```python
from build123d import *

# Parameters (mm, degrees)
F0_R     = 12.7
F0_R_2   = 6.35
F1_DEPTH = 7.62
F0_R_3   = 15.875
F2_DEPTH = 15.24
F3_DEPTH = 27.94
F5_DEPTH = 19.05
F6_DEPTH = 2.54


with BuildPart() as f1:
    # F0 (on Top) → F1 (new body)
    with BuildSketch(Plane.XY):
        Circle(F0_R)
        Circle(F0_R_2, mode=Mode.SUBTRACT)
    extrude(amount=F1_DEPTH)

    # F0 (on Top) → F2 (join)
    with BuildSketch(Plane.XY):
        Circle(F0_R_3)
        Circle(F0_R, mode=Mode.SUBTRACT)
    extrude(amount=F2_DEPTH)

    # F0 (on Top) → F3 (join)
    with BuildSketch(Plane.XY):
        Circle(F0_R_2)
    extrude(amount=F3_DEPTH)

    # F4 (on face) → F5 (join)
    with BuildSketch(Plane.XY.offset(27.94)):
        with BuildLine():
            Line((0, 0), (2.4892, -1.8669))
            ThreePointArc((2.4892, -1.8669), (2.9518280819, -0.983942694), (3.1115, 0))
            ThreePointArc((3.1115, 0), (2.8697186557, 1.2025585587), (2.1819502092, 2.2182257628))
            Line((2.1819502092, 2.2182257628), (0, 0))
        make_face()
        with BuildLine():
            ThreePointArc((2.1819502092, 2.2182257628), (1.6749519392, 2.6222067522), (1.095248, 2.912364))
            Line((1.095248, 2.912364), (0, 0))
            Line((0, 0), (2.1819502092, 2.2182257628))
        make_face()
        with BuildLine():
            ThreePointArc((-2.7755672417, 1.4062925502), (-3.0996598031, -0.2711850936), (-2.4892, -1.8669))
            Line((-2.4892, -1.8669), (0, 0))
            Line((0, 0), (-2.7755672417, 1.4062925502))
        make_face()
        with BuildLine():
            Line((0, 0), (-2.4892, 1.8669))
            ThreePointArc((-2.4892, 1.8669), (-2.6424388986, 1.642847807), (-2.7755672417, 1.4062925502))
            Line((-2.7755672417, 1.4062925502), (0, 0))
        make_face()
        with BuildLine():
            Line((0, 0), (1.095248, 2.912364))
            ThreePointArc((1.095248, 2.912364), (-0.87122, 2.98704), (-2.4892, 1.8669))
            Line((-2.4892, 1.8669), (0, 0))
        make_face()
        with BuildLine():
            ThreePointArc((-2.4892, -1.8669), (0, -3.1115), (2.4892, -1.8669))
            Line((2.4892, -1.8669), (0, 0))
            Line((0, 0), (-2.4892, -1.8669))
        make_face()
    extrude(amount=F5_DEPTH)

    # F4 (on face) → F6 (join)
    with BuildSketch(Plane.XY.offset(27.94)):
        with BuildLine():
            ThreePointArc((-7.2164748284, 3.6563606306), (-8.0591154881, -0.7050812433), (-6.47192, -4.85394))
            Line((-6.47192, -4.85394), (-5.08, -3.81))
            ThreePointArc((-5.08, -3.81), (-6.3258363329, -0.5534389664), (-5.6644229422, 2.8699847964))
            Line((-5.6644229422, 2.8699847964), (-7.2164748284, 3.6563606306))
        make_face()
        with BuildLine():
            Line((-5.08, 3.81), (-6.47192, 4.85394))
            ThreePointArc((-6.47192, 4.85394), (-6.8703411364, 4.2714042983), (-7.2164748284, 3.6563606306))
            Line((-7.2164748284, 3.6563606306), (-5.6644229422, 2.8699847964))
            ThreePointArc((-5.6644229422, 2.8699847964), (-5.3927324462, 3.3527506266), (-5.08, 3.81))
        make_face()
        with BuildLine():
            Line((2.2352, 5.9436), (2.8476448, 7.5721464))
            ThreePointArc((2.8476448, 7.5721464), (-2.265172, 7.766304), (-6.47192, 4.85394))
            Line((-6.47192, 4.85394), (-5.08, 3.81))
            ThreePointArc((-5.08, 3.81), (-1.778, 6.096), (2.2352, 5.9436))
        make_face()
        with BuildLine():
            ThreePointArc((5.6730705438, 5.7673869833), (4.3548750419, 6.8177375558), (2.8476448, 7.5721464))
            Line((2.8476448, 7.5721464), (2.2352, 5.9436))
            ThreePointArc((2.2352, 5.9436), (3.4182692637, 5.3514423515), (4.4529596105, 4.5269913526))
            Line((4.4529596105, 4.5269913526), (5.6730705438, 5.7673869833))
        make_face()
        with BuildLine():
            Line((5.08, -3.81), (6.47192, -4.85394))
            ThreePointArc((6.47192, -4.85394), (7.6747530129, -2.5582510043), (8.0899, 0))
            ThreePointArc((8.0899, 0), (7.4612685048, 3.1266522526), (5.6730705438, 5.7673869833))
            Line((5.6730705438, 5.7673869833), (4.4529596105, 4.5269913526))
            ThreePointArc((4.4529596105, 4.5269913526), (5.8565686851, 2.4542011402), (6.35, 0))
            ThreePointArc((6.35, 0), (6.0241389426, -2.0080463142), (5.08, -3.81))
        make_face()
        with BuildLine():
            ThreePointArc((-6.47192, -4.85394), (0, -8.0899), (6.47192, -4.85394))
            Line((6.47192, -4.85394), (5.08, -3.81))
            ThreePointArc((5.08, -3.81), (0, -6.35), (-5.08, -3.81))
            Line((-5.08, -3.81), (-6.47192, -4.85394))
        make_face()
    extrude(amount=-F6_DEPTH)


solid = f1.part
```
The listing builds one solid part. Answer for the finished solid, in the listing's coordinates (mm). A direction names the side the tool comes from. Round coordinates to 2 decimals unless told otherwise and drop trailing zeros. Loops run counter-clockwise (first coordinate to the right, second up) from the corner with the lowest first, then second, coordinate; pieces in that order, holes last.
Q1. Section C-C, the plane y = 10 is taken. Determine the outline of the cut face in (x, z), then the cut area to 3 significant figures.
Q2. Given pin 1 Ø2 at (x, z) = (6, 10.5) entering from +Y; pin 2 Ø1.5 at (x, z) = (3, 32) entering from -Y; pin 3 Ø4 at (x, y) = (-8.5, -5) entering from -Z; pin 4 Ø1 at (x, y) = (9.5, 7.5) entering from +Z, each flat-ended and moving along its own axis, determine where each tip first touches the part or whether it passes through.
Q3. For a pull along Y with two mould halves and no side action, classify faces 4 (the face through (-3.441, -15.497, 7.513)), 5 (the face through (3, 6, 7.62)), 6 (the face through (0, 0, 46.99)) as released by +Y, released by -Y, zero draft, split by the parting line, or undercut.
Q4. Section A-A, the plane z = 12.5 is taken. Determine the outline of the cut face in (x, y) (3 decimals), then the cut area to 3 significant figures.
Q5. Which of the six approach directions +Z, -Z, +X, -X, +Y, -Y give full straight-line access (tool end or side, diameter ignored) to faces 1 (the face through (0, 0, 0)), 2 (the face through (-2.75, -12.4, 11.38)), 3 (the face through (5.866, -2.432, 16.386))?
Q6. Find the intervals of material crossed by line 1 (Y direction, x = 0, z = 11.5) (3 decimals); line 2 (X direction, y = 4.5, z = 13); line 3 (X direction, y = -5, z = 15), in increasing order.
Q7. Section D-D, the plane z = 37 is taken. Determine the outline of the cut face in (x, y), then the cut area to 3 significant figures.
Completed:
1. outline: (-12.33, 0) - (12.33, 0) - (12.33, 15.24) - (7.83, 15.24) - (7.83, 7.62) - (-7.83, 7.62) - (-7.83, 15.24) - (-12.33, 15.24) - close
1. area: 256 mm2
2. pin 1: stops at y = 15.07
2. pin 2: stops at y = -2.15
2. pin 3: stops at z = 0
2. pin 4: stops at z = 7.62
3. face 4: split by the parting line
3. face 5: undercut
3. face 6: zero draft
4. outline: circle Ø31.75 at (0, 0); circle Ø12.7 at (0, 0); hole circle Ø25.4 at (0, 0)
4. area: 412 mm2
5. face 1: -Z, +X, -X, +Y, -Y
5. face 2: +Z
5. face 3: none
6. line 1: y = -15.875 to -12.7, -6.35 to 6.35, 12.7 to 15.875
6. line 2: x = -15.22 to -11.88, -4.48 to 4.48, 11.88 to 15.22
6. line 3: x = -15.07 to -11.67, -3.91 to 3.91, 11.67 to 15.07
7. outline: circle Ø6.22 at (0, 0)
7. area: 30.4 mm2
